```python
from build123d import *

# Parameters (mm, degrees)
BOSS_EXTRUDE6_DEPTH = 1.6


with BuildPart() as part:
    # Sketch1 → Boss-Extrude6 (new body)
    with BuildSketch(Plane.XY):
        with BuildLine():
            Line((21.906891383, -3.406135598), (106.362891383, -3.406135598))
            ThreePointArc((106.362891383, -3.406135598), (109.191318508, -2.234562723), (110.362891383, 0.593864402))
            Line((110.362891383, 0.593864402), (110.362891383, 76.363864402))
            ThreePointArc((110.362891383, 76.363864402), (109.191318508, 79.192291526), (106.362891383, 80.363864402))
            Line((106.362891383, 80.363864402), (21.906791383, 80.363864402))
            ThreePointArc((21.906791383, 80.363864402), (19.078364258, 79.192291526), (17.906791383, 76.363864402))
            ThreePointArc((17.906791383, 76.363864402), (17.321004945, 74.949650839), (15.906791383, 74.363864402))
            Line((15.906791383, 74.363864402), (0.364791383, 74.363864402))
            ThreePointArc((0.364791383, 74.363864402), (-0.342315398, 74.070971183), (-0.635208617, 73.363864402))
            Line((-0.635208617, 73.363864402), (-0.63368713, 56.102469993))
            ThreePointArc((-0.63368713, 56.102469993), (-0.340793912, 55.395363212), (0.36631287, 55.102469993))
            Line((0.36631287, 55.102469993), (9.26811287, 55.102469993))
            ThreePointArc((9.26811287, 55.102469993), (10.682326432, 54.516683555), (11.26811287, 53.102469993))
            Line((11.26811287, 53.102469993), (11.26811287, 41.868269993))
            ThreePointArc((11.26811287, 41.868269993), (11.400327258, 41.153163772), (11.779489777, 40.532604882))
            Line((11.779489777, 40.532604882), (17.330914678, 34.345440723))
            ThreePointArc((17.330914678, 34.345440723), (17.757303341, 33.700014666), (17.906891383, 32.941064402))
            Line((17.906891383, 32.941064402), (17.906891383, 0.593864402))
            ThreePointArc((17.906891383, 0.593864402), (19.078464258, -2.234562723), (21.906891383, -3.406135598))
        make_face()
    extrude(amount=BOSS_EXTRUDE6_DEPTH)


solid = part.part
```
Geometry check sheet. Reference: the model listing, model coordinates, mm. Coordinates: 2 decimals unless noted, no trailing zeros. Write each loop counter-clockwise with the first axis right and the second up, starting at its lowest first coordinate (ties: lowest second). Pieces come first, ordered by that corner, then holes. Notation, with made-up numbers: M 70,58.5 L 87,58.5 A22 cw 87,78.5 Z; hole C -39,-27 d10. An arc over 180 degrees is marked long. Answer as a JSON object with one key per item and string values.
1. Section check A-A, the plane z = 1. Enter the section's corners in (x, y).
Answers below:
{"outline": "M -0.64,73.36 L -0.63,56.1 A1 ccw 0.37,55.1 L 9.27,55.1 A2 cw 11.27,53.1 L 11.27,41.87 A2 ccw 11.78,40.53 L 17.33,34.35 A2 cw 17.91,32.94 L 17.91,0.59 A4 ccw 21.91,-3.41 L 106.36,-3.41 A4 ccw 110.36,0.59 L 110.36,76.36 A4 ccw 106.36,80.36 L 21.91,80.36 A4 ccw 17.91,76.36 A2 cw 15.91,74.36 L 0.36,74.36 A1 ccw Z"}
2. Section check B-B, the plane y = 48. Enter the section's corners in (x, z).
Answers below:
{"outline": "M 11.27,0 L 110.36,0 L 110.36,1.6 L 11.27,1.6 Z"}
3. Scan lines: L1, parallel to X at y = 29.5, z = 0.4; L2, parallel to X at y = 61, z = 0.5; L3, parallel to Y at x = 8, z = 0.1. Record each from-to range of solid material in increasing order.
Answers below:
{"L1": "x = 17.91 to 110.36", "L2": "x = -0.63 to 110.36", "L3": "y = 55.1 to 74.36"}
4. Go/stop test with a flat-tipped pin: pin 1 Ø0.5 at (x, z) = (2.5, 1) entering from -Y. Record where the tip stops, or that it passes through.
Answers below:
{"pin 1": "stops at y = 55.1"}
5. Section check C-C, the plane x = 13.5. Enter the section's corners in (y, z).
Answers below:
{"outline": "M 38.62,0 L 74.36,0 L 74.36,1.6 L 38.62,1.6 Z"}
